from build123d import *

# Parameters (mm, degrees)
SKETCH_1_R               = 20.5
EXTRUDE_1_DEPTH          = 3
CUT_EXTRUDE_1_REACH      = 31.146
SKETCH_2_R               = 2
PATTERN_CIRCULAR_1_COUNT = 6


with BuildPart() as part:
    # 草圖1 → 填料-伸長1 (new body)
    with BuildSketch(Plane(origin=(0, 0, 0), x_dir=(1, 0, 0), z_dir=(0, 1, 0))):
        with Locations(Location((0, 0, 0), (0, 0, 270))):
            Circle(SKETCH_1_R)
    extrude(amount=EXTRUDE_1_DEPTH)

    # 草圖2 → 除料-伸長1 (cut, up to next)
    with BuildSketch(Plane(origin=(0, 3, 0), x_dir=(1, 0, 0), z_dir=(0, 1, 0)), mode=Mode.PRIVATE) as cut_extrude_1_sk1:
        with Locations(Location((0, 15.5, 0), (0, 0, 270))):
            Circle(SKETCH_2_R)
    cut_extrude_1_tool1 = extrude(cut_extrude_1_sk1.sketch, amount=-CUT_EXTRUDE_1_REACH, mode=Mode.PRIVATE) & part.part
    cut_extrude_1 = cut_extrude_1_tool1.solids().sort_by_distance((0, 3, -15.5))[0]
    add(cut_extrude_1, mode=Mode.SUBTRACT)

    # 環狀複製排列1: 除料-伸長1 ×6 about axis
    pattern_circular_1_axis = Axis((0, 0, 0), (0, 1, 0))
    for i in range(1, PATTERN_CIRCULAR_1_COUNT):
        add(cut_extrude_1.rotate(pattern_circular_1_axis, i * 360 / PATTERN_CIRCULAR_1_COUNT), mode=Mode.SUBTRACT)


solid = part.part
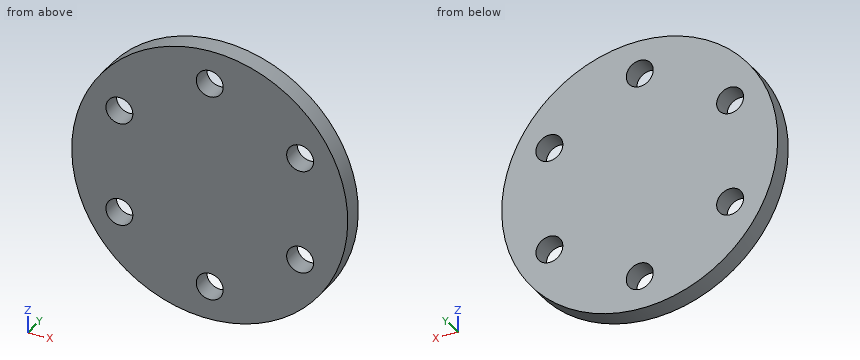
CAD build for the part. Positions are in the model's coordinates, mm. Round coordinates to 2 decimals unless told otherwise and drop trailing zeros. Loops run counter-clockwise (first coordinate to the right, second up) from the corner with the lowest first, then second, coordinate; pieces in that order, holes last. Notation, with made-up numbers: (-2.75, -20.5) - (51.25, -20.5) arc R19 cw to (51.25, 0.5) - close; hole circle Ø5 at (67.5, 7.5). An arc over 180 degrees is marked (long way). Put each result on its own line as item: value.
1. Pin check, flat tips, straight feed: P1, Ø3.5, axis at x = 13.42, z = -7.75, coming from the +Y side; P2, Ø1, axis at x = 10.5, y = 2, coming from the -Z side; P3, Ø1.5, axis at y = 2, z = 7.5, coming from the -X side; P4, Ø1.5, axis at x = -15, y = 2, coming from the -Z side. Stop position of each tip, or through.
Geometry check:
P1: through
P2: z = -17.9
P3: x = -19.36
P4: z = -14.74
2. Slice it at D-D on z = 15.5. List the corners of the cut face in (x, y).
Geometry check:
outline: (-13.42, 0) - (-2, 0) - (-2, 3) - (-13.42, 3) - close; (2, 0) - (13.42, 0) - (13.42, 3) - (2, 3) - close
3. Slice it at C-C on y = 1.15. List the corners of the cut face in (x, z), and give its area (3 significant figures).
Geometry check:
outline: circle Ø41 at (0, 0); hole circle Ø4 at (-13.42, -7.75); hole circle Ø4 at (-13.42, 7.75); hole circle Ø4 at (0, -15.5); hole circle Ø4 at (0, 15.5); hole circle Ø4 at (13.42, -7.75); hole circle Ø4 at (13.42, 7.75)
area: 1,240 mm²
4. Slice it at B-B on z = 7.75. List the corners of the cut face in (x, y), and give its area (3 significant figures).
Geometry check:
outline: (-18.98, 0) - (-15.42, 0) - (-15.42, 3) - (-18.98, 3) - close; (-11.42, 0) - (11.42, 0) - (11.42, 3) - (-11.42, 3) - close; (15.42, 0) - (18.98, 0) - (18.98, 3) - (15.42, 3) - close
area: 89.9 mm²
5. Wall check: line 1 (Z direction, x = -12.5, y = 1.45); line 2 (Z direction, x = -1, y = 1.6); line 3 (X direction, y = 1.15, z = 7.75). Give the ranges that are in metal, low to high.
Geometry check:
line 1: -16.25 to -9.52, -5.98 to 5.98, 9.52 to 16.25
line 2: -20.48 to -17.23, -13.77 to 13.77, 17.23 to 20.48
line 3: -18.98 to -15.42, -11.42 to 11.42, 15.42 to 18.98
6. Slice it at A-A on x = 0. List the corners of the cut face in (y, z).
Geometry check:
outline: (0, -20.5) - (3, -20.5) - (3, -17.5) - (0, -17.5) - close; (0, -13.5) - (3, -13.5) - (3, 13.5) - (0, 13.5) - close; (0, 17.5) - (3, 17.5) - (3, 20.5) - (0, 20.5) - close
